from build123d import *

# Parameters (mm, degrees)
ESQUISSE1_R      = 2.5
ESQUISSE1_R_2    = 2
EXTRUSION1_DEPTH = 8
ESQUISSE2_R      = 4
EXTRUSION2_DEPTH = 4
ESQUISSE3_R      = 2
EXTRUSION3_DEPTH = 15


with BuildPart() as part:
    # Esquisse1 → Extrusion1 (new body)
    with BuildSketch(Plane.XY):
        Polygon((-20, -20), (-20, 15), (-15, 20), (15, 20), (20, 15), (20, -20), align=None)
        Circle(ESQUISSE1_R, mode=Mode.SUBTRACT)
        with Locations((9.899494937, 9.899494937)):
            Circle(ESQUISSE1_R_2, mode=Mode.SUBTRACT)
        with Locations((0, 14)):
            Circle(ESQUISSE1_R_2, mode=Mode.SUBTRACT)
        with Locations((14, 0)):
            Circle(ESQUISSE1_R_2, mode=Mode.SUBTRACT)
        with Locations((9.899494937, -9.899494937)):
            Circle(ESQUISSE1_R_2, mode=Mode.SUBTRACT)
        with Locations((0, -14)):
            Circle(ESQUISSE1_R_2, mode=Mode.SUBTRACT)
        with Locations((-9.899494937, -9.899494937)):
            Circle(ESQUISSE1_R_2, mode=Mode.SUBTRACT)
        with Locations((-14, 0)):
            Circle(ESQUISSE1_R_2, mode=Mode.SUBTRACT)
        with Locations((-9.899494937, 9.899494937)):
            Circle(ESQUISSE1_R_2, mode=Mode.SUBTRACT)
    extrude(amount=EXTRUSION1_DEPTH)

    # Esquisse2 → Extrusion2 (cut)
    with BuildSketch(Plane.XY.offset(8)):
        Circle(ESQUISSE2_R)
    extrude(amount=-EXTRUSION2_DEPTH, mode=Mode.SUBTRACT)

    # Esquisse3 → Extrusion3 (cut)
    with BuildSketch(Plane.XZ.offset(20)):
        with Locations((-15.5, 4)):
            Circle(ESQUISSE3_R)
        with Locations((15.5, 4)):
            Circle(ESQUISSE3_R)
    extrude(amount=-EXTRUSION3_DEPTH, mode=Mode.SUBTRACT)


solid = part.part
CAD build for the part. Positions are in the model's coordinates, mm. A direction names the side the tool comes from. Round coordinates to 2 decimals unless told otherwise and drop trailing zeros. Order: outer loops, then holes, each group sorted by start corner. A loop starts at its lowest first (then second) coordinate and runs counter-clockwise, first axis right, second up. Notation, with made-up numbers: (12, 78.25) -> (50, 78.25) arc R30 ccw to (50, 108.25) -> close; hole circle Ø8 at (-4.75, 2.5). An arc over 180 degrees is marked (long way). Write each question's results on one line, items separated by ' | '.
1. Cut at D-D (z = 7). Count the separate pieces of the cut face and the enclosed holes in it, plus the area to 3 significant figures.
Findings below:
separate pieces: 1 | enclosed holes: 9 | area: 1,420 mm²
2. Cut at B-B (x = 0). Give the cut face in (y, z).
Findings below:
outline: (-20, 0) -> (-16, 0) -> (-16, 8) -> (-20, 8) -> close; (-12, 0) -> (-2.5, 0) -> (-2.5, 4) -> (-4, 4) -> (-4, 8) -> (-12, 8) -> close; (2.5, 0) -> (12, 0) -> (12, 8) -> (4, 8) -> (4, 4) -> (2.5, 4) -> close; (16, 0) -> (20, 0) -> (20, 8) -> (16, 8) -> close
3. Wall check: line 1 along Y through (x, z) = (0, 3.2); line 2 along Y through (x, z) = (0, 6.45); line 3 along Y through (x, z) = (10, 6.5). Give the ranges that are in metal, low to high. Write a range as [from, to].
Findings below:
line 1: y = [-20, -16], [-12, -2.5], [2.5, 12], [16, 20] | line 2: y = [-20, -16], [-12, -4], [4, 12], [16, 20] | line 3: y = [-20, -11.9], [-7.9, 7.9], [11.9, 20]
4. Pull direction Z, two halves, no side cores. Call faces 1 (the face through (0, -4, 0)), 2 (the face through (13.9, -12.6, 2.8)), 3 (the face through (0, -12, 4)): pulls with the +Z half, pulls with the -Z half, needs draft (parallel to the pull), parting line crosses it, or undercut.
Findings below:
face 1: pulls with the -Z half | face 2: undercut | face 3: needs draft
5. Cut at C-C (y = 14). Give the cut face in (x, z), plus the area to 3 significant figures.
Findings below:
outline: (-20, 0) -> (-2, 0) -> (-2, 8) -> (-20, 8) -> close; (2, 0) -> (20, 0) -> (20, 8) -> (2, 8) -> close | area: 288 mm²
6. Flat gauge pins, fed straight in: P1, Ø13, axis at x = 0, y = 0, coming from the -Z side; P2, Ø1.2, axis at x = 15.5, z = 4.5, coming from the -Y side. Where does each tip first touch, or does it go through?
Findings below:
P1: stops at z = 0 | P2: stops at y = -5
7. 3-axis set-ups, long thin cutter, end or side, ignore diameter. For faces 4 (the face through (2, 2, 4)), 5 (the face through (-15.6, -1.2, 3.9)), 6 (the face through (-15.934, -12.605, 2.048)): which of +Z, -Z, +X, -X, +Y, -Y reach the whole face in a straight line?
Findings below:
face 4: +Z | face 5: +Z, -Z | face 6: -Y
8. Cut at A-A (y = -14). Give the cut face in (x, z), plus the area to 3 significant figures.
Findings below:
outline: (-20, 0) -> (-2, 0) -> (-2, 8) -> (-20, 8) -> close; (2, 0) -> (20, 0) -> (20, 8) -> (2, 8) -> close; hole circle Ø4 at (-15.5, 4); hole circle Ø4 at (15.5, 4) | area: 263 mm²
